Check sheet for the modelled part. Datum: model origin and axes. Units: mm. Coordinates: 2 decimals unless noted, no trailing zeros. Write each loop counter-clockwise with the first axis right and the second up, starting at its lowest first coordinate (ties: lowest second). Pieces come first, ordered by that corner, then holes. Notation, with made-up numbers: (24.5, 31.5) - (56.5, 31.5) arc R36 ccw to (56.5, 69.5) - close; hole circle Ø2 at (-30, 86.25). An arc over 180 degrees is marked (long way). Write each question's results on one line, items separated by ' | '.
from build123d import *

# Parameters (mm, degrees)
F1_DEPTH = 2889.25


with BuildPart() as f1:
    # F0 (on Front) → F1 (new body)
    with BuildSketch(Plane.XZ):
        with BuildLine():
            Line((0, 50.8), (0, 0))
            Line((0, 0), (50.8, 0))
            ThreePointArc((50.8, 0), (48.940128, 4.490128), (44.45, 6.35))
            Line((44.45, 6.35), (6.35, 6.35))
            Line((6.35, 6.35), (6.35, 44.45))
            ThreePointArc((6.35, 44.45), (4.490128, 48.940128), (0, 50.8))
        make_face()
    extrude(amount=F1_DEPTH)


solid = f1.part
1. Go/stop test with flat-tipped pins: pin 1 (6 mm diameter, centred on y = -1745, z = 32.5, fed in from -X); pin 2 (2 mm diameter, centred on x = 45, y = -2531.5, fed in from +Z); pin 3 (4 mm diameter, centred on y = -500.5, z = 21, fed in from +X). Record where each tip stops, or that it passes through.
Values follow:
pin 1: stops at x = 0 | pin 2: stops at z = 6.35 | pin 3: stops at x = 6.35
2. Sectioned sample at C-C (z = 15). Record the cut outline in (x, y).
Values follow:
outline: (0, -2889.25) - (6.35, -2889.25) - (6.35, 0) - (0, 0) - close
3. Material ranges on L1, parallel to Z at x = 31, y = -1384.5; L2, parallel to Z at x = 45, y = -1528.5, recorded low to high. Write a range as [from, to].
Values follow:
L1: z = [0, 6.35] | L2: z = [0, 6.33]
4. Sectioned sample at A-A (y = -2572). Record the cut outline in (x, z), then the cut area to 3 significant figures.
Values follow:
outline: (0, 0) - (50.8, 0) arc R6.35 ccw to (44.45, 6.35) - (6.35, 6.35) - (6.35, 44.45) arc R6.35 ccw to (0, 50.8) - close | area: 588 mm^2
5. Sectioned sample at B-B (x = 25). Record the cut outline in (y, z).
Values follow:
outline: (-2889.25, 0) - (0, 0) - (0, 6.35) - (-2889.25, 6.35) - close
